Check sheet for the modelled part. Datum: model origin and axes. Units: mm. Face numbers are marked on the shaded views. A direction names the side the tool comes from. Give positions to 0.01 mm unless a question says otherwise; leave off trailing zeros. Order: outer loops, then holes, each group sorted by start corner. A loop starts at its lowest first (then second) coordinate and runs counter-clockwise, first axis right, second up.
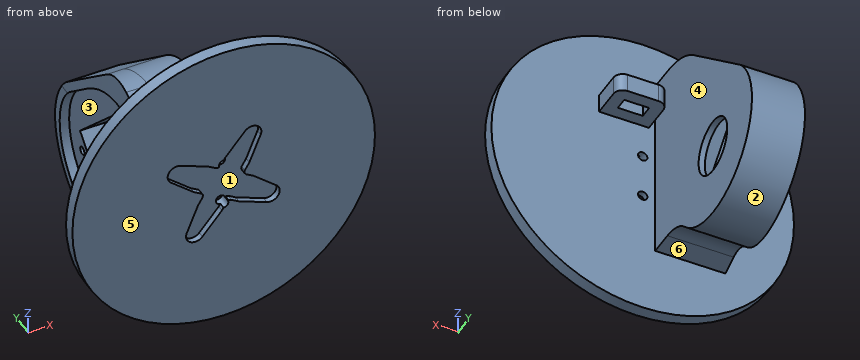
from build123d import *

# Parameters (mm, degrees)
SKETCH2_R                = 48.5
BOSS_EXTRUDE1_DEPTH      = 4
SKETCH4_R                = 1.5
CUT_EXTRUDE2_DEPTH       = 5
SKETCH5_R                = 3.75
CUT_EXTRUDE3_DEPTH       = 1.5
BOSS_EXTRUDE2_DEPTH      = 14
CUT_EXTRUDE5_REACH       = 44.5
SKETCH9_R                = 1.3
CUT_EXTRUDE6_DEPTH       = 7.5
CUT_EXTRUDE9_REACH       = 46.5
SKETCH11_R               = 9
BOSS_EXTRUDE7_DEPTH      = 9
BOSS_EXTRUDE7_DEPTH_BACK = 14
BOSS_EXTRUDE10_DEPTH     = 9
SKETCH27_W               = 16
SKETCH27_H               = 6
BOSS_EXTRUDE11_DEPTH     = 12
FILLET6_R                = 3
CUT_EXTRUDE16_REACH      = 75.05
SKETCH28_W               = 8
SKETCH28_H               = 4
CUT_EXTRUDE17_DEPTH      = 49.5
CUT_EXTRUDE17_DEPTH_BACK = 49.5
CUT_EXTRUDE19_DEPTH      = 2


with BuildPart() as part:
    # Sketch2 → Boss-Extrude1 (new body)
    with BuildSketch(Plane(origin=(0, 0, 0), x_dir=(1, 0, 0), z_dir=(0, 1, 0))):
        Circle(SKETCH2_R)
    extrude(amount=BOSS_EXTRUDE1_DEPTH)

    # Sketch4 → Cut-Extrude2 (cut, through all)
    with BuildSketch(Plane.XZ):
        with Locations((0, 7.25)):
            Circle(SKETCH4_R)
        with Locations((0, -7.25)):
            Circle(SKETCH4_R)
    extrude(amount=-CUT_EXTRUDE2_DEPTH, mode=Mode.SUBTRACT)

    # Sketch5 → Cut-Extrude3 (cut)
    with BuildSketch(Plane.XZ):
        Circle(SKETCH5_R)
    extrude(amount=-CUT_EXTRUDE3_DEPTH, mode=Mode.SUBTRACT)

    # Sketch7 → Boss-Extrude2 (add)
    with BuildSketch(Plane(origin=(-4, 0, 0), x_dir=(0, 0, -1), z_dir=(1, 0, 0))):
        with BuildLine():
            Line((23.129947874, 4), (23.129947874, 11.644549616))
            ThreePointArc((23.129947874, 11.644549616), (24.589048403, 18.743749901), (28.729797284, 24.692011643))
            ThreePointArc((28.729797284, 24.692011643), (29.313383054, 55.284736897), (-1.284289494, 55.479275971))
            Line((-1.284289494, 55.479275971), (-27.227315747, 29.536249718))
            ThreePointArc((-27.227315747, 29.536249718), (-32.64663453, 21.425665997), (-34.549646217, 11.858580188))
            Line((-34.549646217, 11.858580188), (-34.549646217, 4))
            Line((-34.549646217, 4), (23.129947874, 4))
        make_face()
    extrude(amount=-BOSS_EXTRUDE2_DEPTH)

    # Sketch8 → Cut-Extrude5 (cut, up to next)
    with BuildSketch(Plane(origin=(-6, 0, 0), x_dir=(0, 0, -1), z_dir=(1, 0, 0)), mode=Mode.PRIVATE) as cut_extrude5_sk1:
        Polygon((-15.249648422, 25.957567857), (13.741729607, 54.948945886), (28.590972012, 40.099703481), (-0.400406017, 11.108325452), align=None)
    cut_extrude5_tool1 = extrude(cut_extrude5_sk1.sketch, amount=-CUT_EXTRUDE5_REACH, mode=Mode.PRIVATE) & part.part
    add(cut_extrude5_tool1.solids().sort_by_distance((-6, 33.028636, -6.670662))[0], mode=Mode.SUBTRACT)

    # Sketch9 → Cut-Extrude6 (cut)
    with BuildSketch(Plane.ZY.offset(18)):
        with Locations((-20.105690637, 53.534732323)):
            Circle(SKETCH9_R)
        with Locations((-27.176758449, 46.463664511)):
            Circle(SKETCH9_R)
        with Locations((6.764367048, 12.522539014)):
            Circle(SKETCH9_R)
        with Locations((13.83543486, 19.593606826)):
            Circle(SKETCH9_R)
    extrude(amount=-CUT_EXTRUDE6_DEPTH, mode=Mode.SUBTRACT)

    # Sketch11 → Cut-Extrude9 (cut, up to next)
    with BuildSketch(Plane(origin=(-4, 0, 0), x_dir=(0, 0, -1), z_dir=(1, 0, 0)), mode=Mode.PRIVATE) as cut_extrude9_sk1:
        with Locations((13.918506302, 40.276480176)):
            Circle(SKETCH11_R)
    cut_extrude9_tool1 = extrude(cut_extrude9_sk1.sketch, amount=-CUT_EXTRUDE9_REACH, mode=Mode.PRIVATE) & part.part
    add(cut_extrude9_tool1.solids().sort_by_distance((-4, 40.27648, -13.918506))[0], mode=Mode.SUBTRACT)

    # Sketch17 → Boss-Extrude7 (add, two sides)
    with BuildSketch(Plane.ZY.offset(18)) as boss_extrude7_sk:
        with BuildLine():
            ThreePointArc((34.549646217, 11.858580188), (33.008342843, 20.500891953), (28.574482006, 28.077569775))
            ThreePointArc((28.574482006, 28.077569775), (27.915386359, 28.820289685), (27.227315747, 29.536249718))
            Line((27.227315747, 29.536249718), (1.284289494, 55.479275971))
            Line((1.284289494, 55.479275971), (26.295003593, 26.127182305))
            ThreePointArc((26.295003593, 26.127182305), (30.194232218, 19.461281607), (31.549646217, 11.858580188))
            Line((31.549646217, 11.858580188), (31.549646217, 4))
            Line((31.549646217, 4), (34.549646217, 4))
            Line((34.549646217, 4), (34.549646217, 11.858580188))
        make_face()
        with BuildLine():
            Line((28.574482006, 28.077569775), (3.405609837, 57.600596315))
            ThreePointArc((3.405609837, 57.600596315), (-31.461505391, 57.378912253), (-30.796489049, 22.517434639))
            ThreePointArc((-30.796489049, 22.517434639), (-27.345864981, 17.560549854), (-26.129947874, 11.644549616))
            Line((-26.129947874, 11.644549616), (-26.129947874, 4))
            Line((-26.129947874, 4), (-23.129947874, 4))
            Line((-23.129947874, 4), (-23.129947874, 11.644549616))
            ThreePointArc((-23.129947874, 11.644549616), (-24.589048403, 18.743749901), (-28.729797284, 24.692011643))
            ThreePointArc((-28.729797284, 24.692011643), (-29.313383054, 55.284736897), (1.284289494, 55.479275971))
            Line((1.284289494, 55.479275971), (27.227315747, 29.536249718))
            ThreePointArc((27.227315747, 29.536249718), (27.915386359, 28.820289685), (28.574482006, 28.077569775))
        make_face()
    extrude(amount=BOSS_EXTRUDE7_DEPTH)
    extrude(boss_extrude7_sk.sketch, amount=-BOSS_EXTRUDE7_DEPTH_BACK)

    # Sketch25 → Boss-Extrude10 (add)
    with BuildSketch(Plane.ZY.offset(18)):
        with BuildLine():
            ThreePointArc((-28.729797284, 24.692011643), (-24.589048403, 18.743749901), (-23.129947874, 11.644549616))
            Line((-23.129947874, 11.644549616), (-23.129947874, 4))
            Line((-23.129947874, 4), (-15.129947874, 4))
            add(Edge.make_bspline(
                [(-28.729797284, 24.692011643), (-21.954867515, 18.253200081), (-19.09405247, 12.798017691), (-15.129947874, 4)],
                knots=[0, 0, 0, 0, 1, 1, 1, 1], degree=3))
        make_face()
        with BuildLine():
            add(Edge.make_bspline(
                [(11.751619577, 43.19501844), (26.551255916, 25.8264495), (25.549646217, 4)],
                knots=[0, 0, 0, 1, 1, 1], degree=2))
            Line((25.549646217, 4), (31.549646217, 4))
            Line((31.549646217, 4), (31.549646217, 11.858580188))
            ThreePointArc((31.549646217, 11.858580188), (30.194232218, 19.461281607), (26.295003593, 26.127182305))
            Line((26.295003593, 26.127182305), (11.751619577, 43.19501844))
        make_face()
    extrude(amount=BOSS_EXTRUDE10_DEPTH)

    # Sketch27 → Boss-Extrude11 (add)
    with BuildSketch(Plane(origin=(0, 4, 0), x_dir=(1, 0, 0), z_dir=(0, 1, 0))):
        with Locations((6, -21.549646217)):
            Rectangle(SKETCH27_W, SKETCH27_H)
    extrude(amount=BOSS_EXTRUDE11_DEPTH)

    # Fillet6
    fillet6_edges = [part.edges().sort_by_distance(p)[0] for p in [
        (-2, 16, 21.549646217),
        (14, 16, 21.549646217),
    ]]
    fillet(fillet6_edges, radius=FILLET6_R)

    # Sketch28 → Cut-Extrude16 (cut, up to next)
    with BuildSketch(Plane.XY.offset(24.549646217), mode=Mode.PRIVATE) as cut_extrude16_sk1:
        with Locations((6, 10)):
            Rectangle(SKETCH28_W, SKETCH28_H)
    cut_extrude16_tool1 = extrude(cut_extrude16_sk1.sketch, amount=-CUT_EXTRUDE16_REACH, mode=Mode.PRIVATE) & part.part
    add(cut_extrude16_tool1.solids().sort_by_distance((6, 10, 24.549646))[0], mode=Mode.SUBTRACT)

    # Sketch29 → Cut-Extrude17 (cut, two sides)
    with BuildSketch(Plane.XY) as cut_extrude17_sk:
        with BuildLine():
            Line((-21, 64.776480176), (-27, 64.776480176))
            Line((-27, 64.776480176), (-27, 4))
            Line((-27, 4), (-26.5, 4))
            add(Edge.make_bspline(
                [(-21, 64.776480176), (-21.220459696, 34.140901434), (-26.5, 4)],
                knots=[0, 0, 0, 1, 1, 1], degree=2))
        make_face()
    extrude(amount=CUT_EXTRUDE17_DEPTH, mode=Mode.SUBTRACT)
    extrude(cut_extrude17_sk.sketch, amount=-CUT_EXTRUDE17_DEPTH_BACK, mode=Mode.SUBTRACT)

    # Sketch30 → Cut-Extrude19 (cut)
    with BuildSketch(Plane.XZ):
        with BuildLine():
            Line((-1.621331548, 6.623828248), (-2.453034191, 6.751779974))
            Line((-2.453034191, 6.751779974), (-4.898074614, 8.235232927))
            Line((-4.898074614, 8.235232927), (-13.834583132, 11.85774614))
            ThreePointArc((-13.834583132, 11.85774614), (-17.526437212, 10.633625847), (-16.906999469, 6.793762058))
            Line((-16.906999469, 6.793762058), (-9.566495717, 0.540699516))
            Line((-9.566495717, 0.540699516), (-7.121455294, -0.942753437))
            Line((-7.121455294, -0.942753437), (-6.623828248, -1.621331548))
            Line((-6.623828248, -1.621331548), (-6.751779974, -2.453034191))
            Line((-6.751779974, -2.453034191), (-8.235232927, -4.898074614))
            Line((-8.235232927, -4.898074614), (-11.85774614, -13.834583132))
            ThreePointArc((-11.85774614, -13.834583132), (-10.633625847, -17.526437212), (-6.793762058, -16.906999469))
            Line((-6.793762058, -16.906999469), (-0.540699516, -9.566495717))
            Line((-0.540699516, -9.566495717), (0.942753437, -7.121455294))
            Line((0.942753437, -7.121455294), (1.621331548, -6.623828248))
            Line((1.621331548, -6.623828248), (2.453034191, -6.751779974))
            Line((2.453034191, -6.751779974), (4.898074614, -8.235232927))
            Line((4.898074614, -8.235232927), (13.834583132, -11.85774614))
            ThreePointArc((13.834583132, -11.85774614), (17.526437212, -10.633625847), (16.906999469, -6.793762058))
            Line((16.906999469, -6.793762058), (9.566495717, -0.540699516))
            Line((9.566495717, -0.540699516), (7.121455294, 0.942753437))
            Line((7.121455294, 0.942753437), (6.623828248, 1.621331548))
            Line((6.623828248, 1.621331548), (6.751779974, 2.453034191))
            Line((6.751779974, 2.453034191), (8.235232927, 4.898074614))
            Line((8.235232927, 4.898074614), (11.85774614, 13.834583132))
            ThreePointArc((11.85774614, 13.834583132), (10.633625847, 17.526437212), (6.793762058, 16.906999469))
            Line((6.793762058, 16.906999469), (0.540699516, 9.566495717))
            Line((0.540699516, 9.566495717), (-0.942753437, 7.121455294))
            Line((-0.942753437, 7.121455294), (-1.621331548, 6.623828248))
        make_face()
    extrude(amount=-CUT_EXTRUDE19_DEPTH, mode=Mode.SUBTRACT)


solid = part.part
1) Set-up check for the marked faces 1, 2 and 3: record each of +Z, -Z, +X, -X, +Y, -Y from which the full face is reachable in a straight line by a thin tool's end or side.
Recorded:
face 1: -Y
face 2: +X, -X
face 3: -X
2) Section check B-B, the plane x = 26.5. Record the cut outline in (y, z), then the cut area to 3 significant figures.
Recorded:
outline: (0, -40.62) - (4, -40.62) - (4, 40.62) - (0, 40.62) - close
area: 325 mm2
3) Depth check by flat-ended pin: pin 1 Ø1.6 at (y, z) = (19.59, 13.84) entering from -X; pin 2 Ø3 at (y, z) = (12.5, 7) entering from -X; pin 3 Ø6.5 at (y, z) = (8.5, 21.5) entering from +X. Enter the tip coordinate at first touch or a pass-through.
Recorded:
pin 1: stops at x = -10.5
pin 2: stops at x = -18
pin 3: stops at x = 14
4) Section check A-A, the plane x = -33. Record the cut outline in (y, z).
Recorded:
outline: (0, -35.54) - (4, -35.54) - (4, 35.54) - (0, 35.54) - close
5) Draft check along Y on the marked faces 4, 5 and 6. Enter one of: +Y half, -Y half, draft (parallel to the pull), parting line (faces both ways), or undercut.
Recorded:
face 4: draft
face 5: -Y half
face 6: undercut
6) Material ranges on L1, parallel to Z at x = 0, y = 3.25; L2, parallel to X at y = 9, z = 1; L3, parallel to Y at x = 27, z = 39, recorded low to high.
Recorded:
L1: z = -48.5 to -8.75, -5.75 to 5.75, 8.75 to 48.5
L2: x = -18 to -4
L3: y = 0 to 4
